Read the model definition and answer for the solid it produces. Units are mm, in the model's axes. Face numbers are marked on the shaded views. A direction names the side the tool comes from. Round coordinates to 2 decimals unless told otherwise and drop trailing zeros. Write each loop counter-clockwise with the first axis right and the second up, starting at its lowest first coordinate (ties: lowest second). Pieces come first, ordered by that corner, then holes.
from build123d import *

# Parameters (mm, degrees)
SKETCH1_W           = 15
SKETCH1_H           = 30
SKETCH1_R           = 1.5
BOSS_EXTRUDE1_DEPTH = 2
SKETCH3_W           = 15
SKETCH3_H           = 2.034817015
BOSS_EXTRUDE2_DEPTH = 15
SKETCH4_R           = 1.5
CUT_EXTRUDE1_DEPTH  = 15


with BuildPart() as part:
    # Sketch1 → Boss-Extrude1 (new body)
    with BuildSketch(Plane(origin=(0, 0, 0), x_dir=(1, 0, 0), z_dir=(0, 1, 0))):
        with Locations((-21.737545239, 6.883664284)):
            Rectangle(SKETCH1_W, SKETCH1_H)
        with Locations((-21.737545239, 16.883664284)):
            Circle(SKETCH1_R, mode=Mode.SUBTRACT)
        with Locations((-21.737545239, -3.116335716)):
            Circle(SKETCH1_R, mode=Mode.SUBTRACT)
    extrude(amount=BOSS_EXTRUDE1_DEPTH)

    # Sketch3 → Boss-Extrude2 (add)
    with BuildSketch(Plane(origin=(0, 2, 0), x_dir=(1, 0, 0), z_dir=(0, 1, 0))):
        with Locations((-21.737545239, -7.098927209)):
            Rectangle(SKETCH3_W, SKETCH3_H)
    extrude(amount=BOSS_EXTRUDE2_DEPTH)

    # Sketch4 → Cut-Extrude1 (cut)
    with BuildSketch(Plane(origin=(0, 0, 6.081518701), x_dir=(-1, 0, 0), z_dir=(0, 0, -1))):
        with Locations((21.737545239, 9.398162072)):
            Circle(SKETCH4_R)
    extrude(amount=-CUT_EXTRUDE1_DEPTH, mode=Mode.SUBTRACT)


solid = part.part
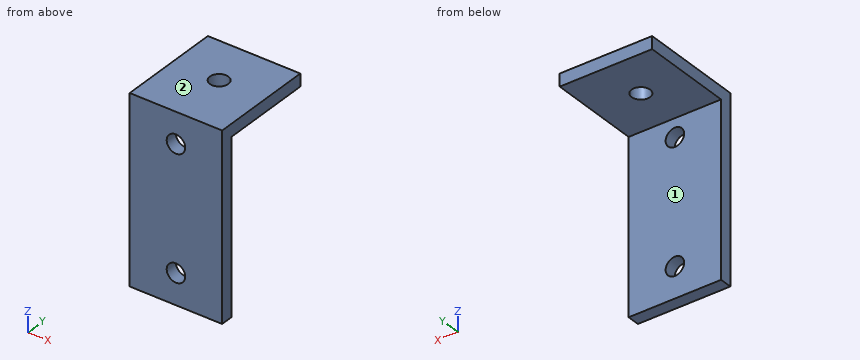
Q1. Section A-A (z = -16) is taken. Determine the outline of the cut face in (x, y), then the cut area to 3 significant figures.
Verdict:
outline: (-29.24, 0) - (-22.95, 0) - (-22.95, 2) - (-29.24, 2) - close; (-20.53, 0) - (-14.24, 0) - (-14.24, 2) - (-20.53, 2) - close
area: 25.2 mm2
Q2. Section D-D (x = -22.5) is taken. Determine the outline of the cut face in (y, z), then the cut area to 3 significant figures.
Verdict:
outline: (0, -21.88) - (2, -21.88) - (2, -18.18) - (0, -18.18) - close; (0, -15.59) - (2, -15.59) - (2, 1.82) - (0, 1.82) - close; (0, 4.41) - (2, 4.41) - (2, 6.08) - (8.11, 6.08) - (8.11, 8.12) - (0, 8.12) - close; (10.69, 6.08) - (17, 6.08) - (17, 8.12) - (10.69, 8.12) - close
area: 74.9 mm2
Q3. Flat-ended cylindrical pins translate along their axes: pin 1 Ø7.5 at (x, z) = (-18, -11) entering from +Y; pin 2 Ø8 at (x, y) = (-21, 10) entering from -Z; pin 3 Ø2.5 at (x, z) = (-21.74, -16.88) entering from +Y. Find the tip coordinate at first contact, or state that the pin passes through.
Verdict:
pin 1: stops at y = 2
pin 2: stops at z = 6.08
pin 3: passes through
Q4. Which of the six approach directions +Z, -Z, +X, -X, +Y, -Y give full straight-line access (tool end or side, diameter ignored) to the marked faces 1 and 2?
Verdict:
face 1: -Z, +X, -X, +Y
face 2: +Z, +X, -X, +Y, -Y
Q5. Straight lines are drawn through the part: probe 1 along Z at (x, y) = (-16.25, 6); probe 2 along Y at (x, z) = (-20.5, -15). For each, find the intervals that lie inside material, in ascending order.
Verdict:
probe 1: z = 6.08 to 8.12
probe 2: y = 0 to 2
Q6. Section B-B (x = -21) is taken. Determine the outline of the cut face in (y, z), then the cut area to 3 significant figures.
Verdict:
outline: (0, -21.88) - (2, -21.88) - (2, -18.19) - (0, -18.19) - close; (0, -15.58) - (2, -15.58) - (2, 1.81) - (0, 1.81) - close; (0, 4.42) - (2, 4.42) - (2, 6.08) - (8.09, 6.08) - (8.09, 8.12) - (0, 8.12) - close; (10.7, 6.08) - (17, 6.08) - (17, 8.12) - (10.7, 8.12) - close
area: 74.8 mm2
Q7. Section C-C (y = 10) is taken. Determine the outline of the cut face in (x, z), then the cut area to 3 significant figures.
Verdict:
outline: (-29.24, 6.08) - (-23.11, 6.08) - (-23.11, 8.12) - (-29.24, 8.12) - close; (-20.36, 6.08) - (-14.24, 6.08) - (-14.24, 8.12) - (-20.36, 8.12) - close
area: 24.9 mm2
